```python
from build123d import *

# Parameters (mm, degrees)
F0_R      = 35
F1_DEPTH  = 30
F2_T      = -4
F3_R      = 5
F5_R      = 5
F7_R      = 8
F7_R_2    = 5
F8_DEPTH  = 80
F9_R      = 5.0065220345
F10_DEPTH = 7
F11_SIZE  = 2
F14_DEPTH = 6.5
F15_R     = 5
F17_R     = 35
F17_R_2   = 33
F18_DEPTH = 3.5
F19_R     = 3
F20_R     = 1.7097163671
F21_DEPTH = 37.001


# Not quite as in the source:
# - a fillet or chamfer that OpenCascade refuses, or shapes differently, is made with other operations: its cross-section is extruded or revolved along the edge and cut away or added


with BuildPart() as f1:
    # F0 (on Front) → F1 (new body)
    with BuildSketch(Plane.XZ):
        Circle(F0_R)
    extrude(amount=F1_DEPTH)

    # F2
    f2_openings = [f1.faces().sort_by_distance(p)[0] for p in [
        (0, -30, 0),
    ]]
    offset(amount=F2_T, openings=f2_openings)

    # F3
    f3_edges = [f1.edges().sort_by_distance(p)[0] for p in [
        (-35, 0, 0),
    ]]
    fillet(f3_edges, radius=F3_R)

    # F5 (on offset) → F6 (join, up to the next surface of F1)
    with BuildSketch(Plane.YZ.offset(47)):
        with Locations((-6.4707305679, 0)):
            Circle(F5_R)
    extrude(until=Until.NEXT, dir=(-1, 0, 0))

    # F7 (on face) → F8 (join)
    with BuildSketch(Plane.YZ.offset(47)):
        with Locations((-6.4707305679, 0)):
            Circle(F7_R)
        with Locations((-6.4707305679, 0)):
            Circle(F7_R_2, mode=Mode.SUBTRACT)
        with Locations((-6.4707305679, 0)):
            Circle(F7_R_2)
    extrude(amount=F8_DEPTH)

    # F9 (on face) → F10 (join)
    with BuildSketch(Plane(origin=(0, 0, 0), x_dir=(-1, 0, 0), z_dir=(0, 1, 0))):
        Circle(F9_R)
    extrude(amount=F10_DEPTH)

    # F11
    f11_edges = [f1.edges().sort_by_distance(p)[0] for p in [
        (5.006522, 7, 0),
    ]]
    chamfer(f11_edges, length=F11_SIZE)

    # F13 (on offset) → F14 (join)
    with BuildSketch(Plane.XZ.offset(26.5)):
        with BuildLine():
            Line((-12, -39.5), (12, -39.5))
            Line((12, -39.5), (12, -32.8785644455))
            ThreePointArc((12, -32.8785644455), (0, -35), (-12, -32.8785644455))
            Line((-12, -32.8785644455), (-12, -39.5))
        make_face()
        with BuildLine():
            ThreePointArc((-12, 32.8785644455), (0, 35), (12, 32.8785644455))
            Line((12, 32.8785644455), (12, 39.5))
            Line((12, 39.5), (-12, 39.5))
            Line((-12, 39.5), (-12, 32.8785644455))
        make_face()
    extrude(amount=-F14_DEPTH)

    # F15
    f15_edges = [f1.edges().sort_by_distance(p)[0] for p in [
        (127, -14.470731, 0),
    ]]
    fillet(f15_edges, radius=F15_R)

    # F16: fillet of radius 5 on 1 edges, made by hand

    # F16_s1 → F16_t2 (revolve, cut)
    with BuildSketch(Plane.XY):
        with BuildLine():
            ThreePointArc((51.582575695, 1.5292694321), (48.8439629074, 0.7125695648), (47, -1.4707305679))
            Line((47, -1.4707305679), (47, 1.5292694321))
            Line((47, 1.5292694321), (51.582575695, 1.5292694321))
        make_face()
    revolve(axis=Axis((47, -6.4707305679, 0), (1, 0, 0)), mode=Mode.SUBTRACT)

    # F17 (on face) → F18 (cut, through all)
    with BuildSketch(Plane.XZ.offset(30)):
        Circle(F17_R)
        Circle(F17_R_2, mode=Mode.SUBTRACT)
    extrude(amount=-F18_DEPTH, mode=Mode.SUBTRACT)

    # F19
    f19_edges = [f1.edges().sort_by_distance(p)[0] for p in [
        (12, -23.25, 39.5),
        (-12, -23.25, 39.5),
        (-12, -23.25, -39.5),
        (12, -23.25, -39.5),
    ]]
    fillet(f19_edges, radius=F19_R)

    # F20 (on face) → F21 (cut, through all)
    with BuildSketch(Plane(origin=(0, 7, 0), x_dir=(-1, 0, 0), z_dir=(0, 1, 0))):
        Circle(F20_R)
    extrude(amount=-F21_DEPTH, mode=Mode.SUBTRACT)


solid = f1.part
```
Work out the finished part from the listing and answer in its coordinate system (mm). A direction names the side the tool comes from. Round coordinates to 2 decimals unless told otherwise and drop trailing zeros. Write each loop counter-clockwise with the first axis right and the second up, starting at its lowest first coordinate (ties: lowest second). Pieces come first, ordered by that corner, then holes. Notation, with made-up numbers: (-2, 31.5) - (42, 31.5) arc R14 cw to (42, 35.5) - close; hole circle Ø3 at (54.25, 51.25). An arc over 180 degrees is marked (long way). Return JSON: item names as keys, results as strings. Group by question number.
Q1. Find the intervals of material crossed by L1, parallel to X at y = -17.25, z = 0; L2, parallel to X at y = -12.5, z = 0; L3, parallel to X at y = -19, z = -10.5, in increasing order.
Q2. The part is cut by section A-A on x = 0. Write down the section's boundary in (y, z).
Q3. The mould has two halves that part along Z. Classify faces 1 (the flat face through (0, 7, -2)), 2 (the cylindrical face through (86.3, 0.92, -3.06)), 3 (the cylindrical face through (-11.14, -23.2, 38.6)), 4 (the flat face through (0, -4, -6)): released by +Z, released by -Z, zero draft, split by the parting line, or undercut.
Q4. Each of these flat-tipped pins is pushed along its axis until it touches: pin 1 Ø10 at (x, z) = (-16.5, -22.5) entering from +Y; pin 2 Ø5.5 at (x, z) = (-4.5, 35) entering from +Y; pin 3 Ø8 at (x, y) = (-7.5, -11) entering from -Z. Where does it stop, or does it pass through?
Q5. For faces 5 (the flat face through (12, -23, -35)), 6 (the cylindrical face through (40.365, -1.852, -1.915)), 7 (the flat face through (-12, -23, -35)), determine the directions among +Z, -Z, +X, -X, +Y, -Y from which every point of the face is accessible in a straight line to the end or side of a thin tool.
Q6. The part is cut by section B-B on x = 96. Write down the section's boundary in (y, z), then the cut area to 3 significant figures.
Solved:
{
 "1": {"L1": "-35 to -31, 31 to 35", "L2": "-35 to -31, 31 to 35, 47.6 to 125.98", "L3": "-33.39 to -29.17, 29.17 to 33.39"},
 "2": {"outline": "(-30, -33) - (-26.5, -33) - (-26.5, -39.5) - (-20, -39.5) - (-20, -35) - (-5, -35) arc R5 ccw to (0, -30) - (0, -5.01) - (5, -5.01) - (7, -3.01) - (7, -1.71) - (-4, -1.71) - (-4, -31) - (-30, -31) - close; (-30, 31) - (-4, 31) - (-4, 1.71) - (7, 1.71) - (7, 3.01) - (5, 5.01) - (0, 5.01) - (0, 30) arc R5 ccw to (-5, 35) - (-20, 35) - (-20, 39.5) - (-26.5, 39.5) - (-26.5, 33) - (-30, 33) - close"},
 "3": {"face 1": "zero draft", "face 2": "split by the parting line", "face 3": "released by +Z", "face 4": "undercut"},
 "4": {"pin 1": "y = 0", "pin 2": "y = -0.69", "pin 3": "z = -34.82"},
 "5": {"face 5": "-Z, +X, +Y, -Y", "face 6": "none", "face 7": "-Z, -X, +Y, -Y"},
 "6": {"outline": "circle Ø16 at (-6.47, 0)", "area": "201 mm²"}
}
